Can you work these out from the model? Positions are in its coordinate system, mm. A direction names the side the tool comes from. Give positions to 0.01 mm unless a question says otherwise; leave off trailing zeros. Loops run counter-clockwise (first coordinate to the right, second up) from the corner with the lowest first, then second, coordinate; pieces in that order, holes last. Notation, with made-up numbers: (3.25, 73) - (15.25, 73) arc R28 ccw to (15.25, 94) - close; hole circle Ø5 at (1, 79.25). An arc over 180 degrees is marked (long way). Answer as a JSON object with one key per item and string values.
```python
from build123d import *

# Parameters (mm, degrees)
EXTRUDE_2_DEPTH = 20
EXTRUDE_3_DEPTH = 15
EXTRUDE_4_DEPTH = 10
EXTRUDE_5_DEPTH = 5


with BuildPart() as part:
    # Sketch 1 → Extrude 2 (new body)
    with BuildSketch(Plane(origin=(0, 0, 0), x_dir=(1, 0, 0), z_dir=(0, 1, 0))):
        Polygon((-12.5, -10), (-7.5, -10), (-7.5, -5), (-7.5, 0), (-7.5, 5), (-2.5, 5), (2.5, 5), (12.5, 5), (12.5, 10), (-12.5, 10), align=None)
        Polygon((-7.5, 5), (-7.5, 0), (-2.5, 5), align=None)
    extrude(amount=EXTRUDE_2_DEPTH)

    # Sketch 1_4 → Extrude 3 (add)
    with BuildSketch(Plane(origin=(0, 0, 0), x_dir=(1, 0, 0), z_dir=(0, 1, 0))):
        Polygon((-7.5, 0), (-7.5, -5), (2.5, 5), (-2.5, 5), align=None)
    extrude(amount=EXTRUDE_3_DEPTH)

    # Sketch 1_5 → Extrude 4 (add)
    with BuildSketch(Plane(origin=(0, 0, 0), x_dir=(1, 0, 0), z_dir=(0, 1, 0))):
        Polygon((-7.5, -5), (-7.5, -10), (2.5, 0), (12.5, -10), (12.5, 5), (2.5, 5), align=None)
    extrude(amount=EXTRUDE_4_DEPTH)

    # Sketch 1_6 → Extrude 5 (add)
    with BuildSketch(Plane(origin=(0, 0, 0), x_dir=(1, 0, 0), z_dir=(0, 1, 0))):
        Polygon((2.5, 0), (-7.5, -10), (12.5, -10), align=None)
    extrude(amount=EXTRUDE_5_DEPTH)


solid = part.part
```
1) Imagine slicing it at D-D on x = 5.25. Write out the boundary of the cut face in (y, z).
Check sheet entries:
{"outline": "(0, -10) - (20, -10) - (20, -5) - (10, -5) - (10, 2.75) - (5, 2.75) - (5, 10) - (0, 10) - close"}
2) Imagine slicing it at A-A on x = -0.5. Write out the boundary of the cut face in (y, z).
Check sheet entries:
{"outline": "(0, -10) - (20, -10) - (20, -5) - (15, -5) - (15, -2) - (10, -2) - (10, 3) - (5, 3) - (5, 10) - (0, 10) - close"}
3) If we mould it in two halves opening along X, with no side actions, what happens to faces 1 (the flat face through (-7.5, 16, 6)), 2 (the flat face through (7, 15, -5)), 3 (the flat face through (7.4, 7.5, 4.9))? For each: released by +X, released by -X, zero draft, split by the parting line, or undercut.
Check sheet entries:
{"face 1": "released by +X", "face 2": "zero draft", "face 3": "undercut"}
4) Imagine slicing it at B-B on y = 18. Write out the boundary of the cut face in (x, z).
Check sheet entries:
{"outline": "(-12.5, -10) - (12.5, -10) - (12.5, -5) - (-2.5, -5) - (-7.5, 0) - (-7.5, 10) - (-12.5, 10) - close"}
5) Which directions (+Z, -Z, +X, -X, +Y, -Y) give clear straight access to the entire face, cutting with the end or side of a thin tool? Please do faces 4 (the flat face through (0, 0, 0)), 5 (the flat face through (-2.6, 12.5, 0.1)), 6 (the flat face through (2, 5, 6)).
Check sheet entries:
{"face 4": "+Z, -Z, +X, -X, -Y", "face 5": "+Z, +X, +Y", "face 6": "+Z, +Y"}
6) Imagine slicing it at C-C on z = 3.75. Write out the boundary of the cut face in (x, y), and give its area (3 significant figures).
Check sheet entries:
{"outline": "(-12.5, 0) - (12.5, 0) - (12.5, 10) - (6.25, 10) - (6.25, 5) - (-1.25, 5) - (-1.25, 10) - (-6.25, 10) - (-6.25, 15) - (-7.5, 15) - (-7.5, 20) - (-12.5, 20) - close", "area": "269 mm2"}
7) I'm going to push flat-ended pins straight in: P1, Ø10, axis at x = 3.5, z = 4, coming from the +Y side; P2, Ø5, axis at x = 4, y = 17.5, coming from the +Z side; P3, Ø12, axis at x = -1, z = 4, coming from the +Y side. Where does each tip first touch, or does it pass through?
Check sheet entries:
{"P1": "y = 10", "P2": "z = -5", "P3": "y = 15"}
8) I need wall thicknesses on L1, parallel to Y at x = 9.5, z = 6.5; L2, parallel to Z at x = 10, y = 15; L3, parallel to Y at x = -7, z = 3.5. Which ranges of each line are inside material? Lowest first, please.
Check sheet entries:
{"L1": "0 to 10", "L2": "-10 to -5", "L3": "0 to 15"}
